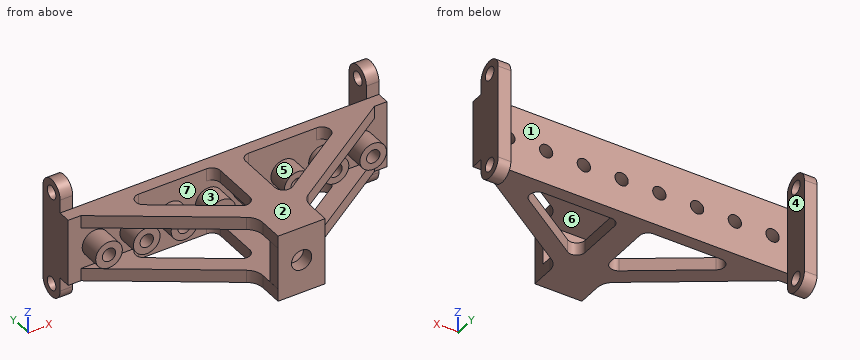
```python
from build123d import *

# Parameters (mm, degrees)
SKETCH1_W            = 70
SKETCH1_H            = 16
SKETCH1_R            = 1.5875
BOSS_EXTRUDE1_DEPTH  = 3
BOSS_EXTRUDE6_DEPTH  = 3
BOSS_EXTRUDE9_START  = -3
BOSS_EXTRUDE9_DEPTH  = 3
SKETCH7_W            = 11.213160903
SKETCH7_H            = 16
SKETCH7_R            = 2.413
BOSS_EXTRUDE10_DEPTH = 3
SKETCH10_R           = 1.5875
BOSS_EXTRUDE11_DEPTH = 3
BOSS_EXTRUDE12_START = 3
SKETCH11_R           = 1.5875
BOSS_EXTRUDE12_DEPTH = 3
SKETCH12_R           = 3.175
SKETCH12_R_2         = 1.5875
BOSS_EXTRUDE13_DEPTH = 5


with BuildPart() as part:
    # Sketch1 → Boss-Extrude1 (new body)
    with BuildSketch(Plane(origin=(0, 0, 0), x_dir=(1, 0, 0), z_dir=(0, 1, 0))):
        Rectangle(SKETCH1_W, SKETCH1_H)
        with Locations(Location((-4.5, 0, 0), (0, 0, 270))):
            Circle(SKETCH1_R, mode=Mode.SUBTRACT)
        with Locations(Location((4.5, 0, 0), (0, 0, 270))):
            Circle(SKETCH1_R, mode=Mode.SUBTRACT)
        with Locations(Location((13.5, 0, 0), (0, 0, 270))):
            Circle(SKETCH1_R, mode=Mode.SUBTRACT)
        with Locations(Location((22.5, 0, 0), (0, 0, 270))):
            Circle(SKETCH1_R, mode=Mode.SUBTRACT)
        with Locations(Location((31.5, 0, 0), (0, 0, 270))):
            Circle(SKETCH1_R, mode=Mode.SUBTRACT)
        with Locations(Location((-13.5, 0, 0), (0, 0, 270))):
            Circle(SKETCH1_R, mode=Mode.SUBTRACT)
        with Locations(Location((-22.5, 0, 0), (0, 0, 270))):
            Circle(SKETCH1_R, mode=Mode.SUBTRACT)
        with Locations(Location((-31.5, 0, 0), (0, 0, 270))):
            Circle(SKETCH1_R, mode=Mode.SUBTRACT)
    extrude(amount=-BOSS_EXTRUDE1_DEPTH)

    # Sketch3 → Boss-Extrude6 (add)
    with BuildSketch(Plane(origin=(0, 0, -8), x_dir=(-1, 0, 0), z_dir=(0, 0, -1))):
        with BuildLine():
            ThreePointArc((-7.390034655, -21.480696382), (-6.086556875, -22.920616292), (-5.615003916, -24.804776975))
            Line((-5.615003916, -24.804776975), (-5.615003916, -30.4))
            Line((-5.615003916, -30.4), (5.615003916, -30.4))
            Line((5.615003916, -30.4), (5.615003916, -24.804776975))
            ThreePointArc((5.615003916, -24.804776975), (6.086556875, -22.920616292), (7.390034655, -21.480696382))
            Line((7.390034655, -21.480696382), (35, -3))
            Line((35, -3), (35, 0))
            Line((35, 0), (-35, 0))
            Line((-35, 0), (-35, -3))
            Line((-35, -3), (-7.390034655, -21.480696382))
        make_face()
        with BuildLine():
            Line((-6.11248463, -17.522461887), (-22.337839864, -6.662040296))
            ThreePointArc((-22.337839864, -6.662040296), (-23.139001046, -4.418656983), (-21.225355233, -3))
            Line((-21.225355233, -3), (-5, -3))
            ThreePointArc((-5, -3), (-3.585786438, -3.585786438), (-3, -5))
            Line((-3, -5), (-3, -15.860421591))
            ThreePointArc((-3, -15.860421591), (-4.057919659, -17.624645111), (-6.11248463, -17.522461887))
        make_face(mode=Mode.SUBTRACT)
        with BuildLine():
            Line((3, -15.860421591), (3, -5))
            ThreePointArc((3, -5), (3.585786438, -3.585786438), (5, -3))
            Line((5, -3), (21.225355233, -3))
            ThreePointArc((21.225355233, -3), (23.139001046, -4.418656983), (22.337839864, -6.662040296))
            Line((22.337839864, -6.662040296), (6.11248463, -17.522461887))
            ThreePointArc((6.11248463, -17.522461887), (4.057919659, -17.624645111), (3, -15.860421591))
        make_face(mode=Mode.SUBTRACT)
    extrude(amount=-BOSS_EXTRUDE6_DEPTH)

    # Sketch6 → Boss-Extrude9 (add)
    with BuildSketch(Plane.XY.offset(8).offset(BOSS_EXTRUDE9_START)):
        with BuildLine():
            ThreePointArc((-7.390034655, -21.480696382), (-6.086556875, -22.920616292), (-5.615003916, -24.804776975))
            Line((-5.615003916, -24.804776975), (-5.615003916, -30.4))
            Line((-5.615003916, -30.4), (5.615003916, -30.4))
            Line((5.615003916, -30.4), (5.615003916, -24.804776975))
            ThreePointArc((5.615003916, -24.804776975), (6.086556875, -22.920616292), (7.390034655, -21.480696382))
            Line((7.390034655, -21.480696382), (35, -3))
            Line((35, -3), (35, 0))
            Line((35, 0), (-35, 0))
            Line((-35, 0), (-35, -3))
            Line((-35, -3), (-7.390034655, -21.480696382))
        make_face()
        with BuildLine():
            Line((-6.11248463, -17.522461887), (-22.337839864, -6.662040296))
            ThreePointArc((-22.337839864, -6.662040296), (-23.139001046, -4.418656983), (-21.225355233, -3))
            Line((-21.225355233, -3), (-5, -3))
            ThreePointArc((-5, -3), (-3.585786438, -3.585786438), (-3, -5))
            Line((-3, -5), (-3, -15.860421591))
            ThreePointArc((-3, -15.860421591), (-4.057919659, -17.624645111), (-6.11248463, -17.522461887))
        make_face(mode=Mode.SUBTRACT)
        with BuildLine():
            Line((3, -15.860421591), (3, -5))
            ThreePointArc((3, -5), (3.585786438, -3.585786438), (5, -3))
            Line((5, -3), (21.225355233, -3))
            ThreePointArc((21.225355233, -3), (23.139001046, -4.418656983), (22.337839864, -6.662040296))
            Line((22.337839864, -6.662040296), (6.11248463, -17.522461887))
            ThreePointArc((6.11248463, -17.522461887), (4.057919659, -17.624645111), (3, -15.860421591))
        make_face(mode=Mode.SUBTRACT)
    extrude(amount=BOSS_EXTRUDE9_DEPTH)

    # Sketch7 → Boss-Extrude10 (add)
    with BuildSketch(Plane.XZ.offset(30.4)):
        with Locations((0.008423464, 0)):
            Rectangle(SKETCH7_W, SKETCH7_H)
        Circle(SKETCH7_R, mode=Mode.SUBTRACT)
    extrude(amount=-BOSS_EXTRUDE10_DEPTH)

    # Sketch10 → Boss-Extrude11 (add)
    with BuildSketch(Plane(origin=(35, 0, 0), x_dir=(0, 0, -1), z_dir=(1, 0, 0))):
        with BuildLine():
            Line((-11.175, 0), (-8, 0))
            Line((-8, 0), (-8, -3))
            Line((-8, -3), (8, -3))
            Line((8, -3), (8, 0))
            Line((8, 0), (11.175, 0))
            ThreePointArc((11.175, 0), (14.35, 3.175), (11.175, 6.35))
            Line((11.175, 6.35), (-11.175, 6.35))
            ThreePointArc((-11.175, 6.35), (-14.35, 3.175), (-11.175, 0))
        make_face()
        with Locations(Location((11.175, 3.175, 0), (0, 0, 180))):
            Circle(SKETCH10_R, mode=Mode.SUBTRACT)
        with Locations((-11.175, 3.175)):
            Circle(SKETCH10_R, mode=Mode.SUBTRACT)
    extrude(amount=BOSS_EXTRUDE11_DEPTH)

    # Sketch11 → Boss-Extrude12 (add)
    with BuildSketch(Plane.ZY.offset(35).offset(BOSS_EXTRUDE12_START)):
        with BuildLine():
            Line((-11.175, 0), (-8, 0))
            Line((-8, 0), (-8, -3))
            Line((-8, -3), (8, -3))
            Line((8, -3), (8, 0))
            Line((8, 0), (11.175, 0))
            ThreePointArc((11.175, 0), (14.35, 3.175), (11.175, 6.35))
            Line((11.175, 6.35), (-11.175, 6.35))
            ThreePointArc((-11.175, 6.35), (-14.35, 3.175), (-11.175, 0))
        make_face()
        with Locations(Location((11.175, 3.175, 0), (0, 0, 180))):
            Circle(SKETCH11_R, mode=Mode.SUBTRACT)
        with Locations((-11.175, 3.175)):
            Circle(SKETCH11_R, mode=Mode.SUBTRACT)
    extrude(amount=-BOSS_EXTRUDE12_DEPTH)

    # Sketch12 → Boss-Extrude13 (add)
    # profile 1 of 8: a face of its own
    with BuildSketch(Plane.XZ.offset(3)):
        with Locations(Location((-31.5, 0, 0), (0, 0, 270))):
            Circle(SKETCH12_R)
        with Locations(Location((-31.5, 0, 0), (0, 0, 90))):
            Circle(SKETCH12_R_2, mode=Mode.SUBTRACT)
    # profile 2 of 8: a face of its own
    with BuildSketch(Plane.XZ.offset(3)):
        with Locations(Location((-22.5, 0, 0), (0, 0, 270))):
            Circle(SKETCH12_R)
        with Locations(Location((-22.5, 0, 0), (0, 0, 90))):
            Circle(SKETCH12_R_2, mode=Mode.SUBTRACT)
    # profile 3 of 8: a face of its own
    with BuildSketch(Plane.XZ.offset(3)):
        with Locations(Location((-13.5, 0, 0), (0, 0, 270))):
            Circle(SKETCH12_R)
        with Locations(Location((-13.5, 0, 0), (0, 0, 90))):
            Circle(SKETCH12_R_2, mode=Mode.SUBTRACT)
    # profile 4 of 8: a face of its own
    with BuildSketch(Plane.XZ.offset(3)):
        with Locations(Location((-4.5, 0, 0), (0, 0, 270))):
            Circle(SKETCH12_R)
        with Locations(Location((-4.5, 0, 0), (0, 0, 90))):
            Circle(SKETCH12_R_2, mode=Mode.SUBTRACT)
    # profile 5 of 8: a face of its own
    with BuildSketch(Plane.XZ.offset(3)):
        with Locations(Location((4.5, 0, 0), (0, 0, 270))):
            Circle(SKETCH12_R)
        with Locations(Location((4.5, 0, 0), (0, 0, 90))):
            Circle(SKETCH12_R_2, mode=Mode.SUBTRACT)
    # profile 6 of 8: a face of its own
    with BuildSketch(Plane.XZ.offset(3)):
        with Locations(Location((13.5, 0, 0), (0, 0, 270))):
            Circle(SKETCH12_R)
        with Locations(Location((13.5, 0, 0), (0, 0, 90))):
            Circle(SKETCH12_R_2, mode=Mode.SUBTRACT)
    # profile 7 of 8: a face of its own
    with BuildSketch(Plane.XZ.offset(3)):
        with Locations(Location((22.5, 0, 0), (0, 0, 270))):
            Circle(SKETCH12_R)
        with Locations(Location((22.5, 0, 0), (0, 0, 90))):
            Circle(SKETCH12_R_2, mode=Mode.SUBTRACT)
    # profile 8 of 8: a face of its own
    with BuildSketch(Plane.XZ.offset(3)):
        with Locations(Location((31.5, 0, 0), (0, 0, 270))):
            Circle(SKETCH12_R)
        with Locations(Location((31.5, 0, 0), (0, 0, 90))):
            Circle(SKETCH12_R_2, mode=Mode.SUBTRACT)
    extrude(amount=BOSS_EXTRUDE13_DEPTH)


solid = part.part
```
Design review of the part built by this model. Coordinates are the model's own, in mm. Face numbers are marked on the shaded views. A direction names the side the tool comes from. Coordinates: 2 decimals unless noted, no trailing zeros. Order: outer loops, then holes, each group sorted by start corner. A loop starts at its lowest first (then second) coordinate and runs counter-clockwise, first axis right, second up. Notation, with made-up numbers: (57, -28) -> (72, -28) arc R25 ccw to (72, -7) -> close; hole circle Ø8 at (-25.75, 81). An arc over 180 degrees is marked (long way). One line per item, written item: value. Start each with the question number.
Q1. Take a section at B-B, the plane x = 31.5. State the section outline as (y, z) points (1 decimal).
Q2. Insertion check: pin 1 Ø10 at (x, y) = (-3.5, -0.5) entering from -Z; pin 2 Ø2.5 at (x, z) = (-4.5, 0) entering from +Y; pin 3 Ø6 at (x, y) = (22.5, -17.5) entering from -Z; pin 4 Ø6 at (x, z) = (16.5, 1) entering from +Y. Each pin has a flat end and moves straight along its axis. Give the tip position at first contact, or say it passes through.
Q3. For probe 1 along X at (y, z) = (5.5, -7.75); probe 2 along Y at (x, z) = (12, -3.25); probe 3 along Z at (x, y) = (-31, -4), list the stretches that pass through material, from the lowest coordinate up.
Q4. Take a section at A-A, the plane z = -7. State the section outline as (x, y) points (3 decimals), then the cut area to 3 significant figures.
Q5. Mouldability with a two-part tool opening along Y and no side actions: class the marked faces 1, 2 and 3 as pulls with the +Y half, pulls with the -Y half, needs draft (parallel to the pull), parting line crosses it, or undercut.
Q6. Tool access review of the marked faces 4, 5, 6 and 7: name each direction out of +Z, -Z, +X, -X, +Y, -Y from which nothing blocks a thin tool from reaching the whole face with its end or side.
Q7. Take a section at C-C, the plane y = -1. Give the number of separate pieces and of enclosed holes in the cut face, then the cut area to 3 significant figures.
Values follow:
1. outline: (-8, -3.2) -> (-3, -3.2) -> (-3, -5) -> (-5.3, -5) -> (-5.3, -8) -> (0, -8) -> (0, -1.6) -> (-8, -1.6) -> close; (-8, 1.6) -> (0, 1.6) -> (0, 8) -> (-5.3, 8) -> (-5.3, 5) -> (-3, 5) -> (-3, 3.2) -> (-8, 3.2) -> close
2. pin 1: stops at z = -8
2. pin 2: stops at y = -27.4
2. pin 3: passes through
2. pin 4: stops at y = 0
3. probe 1: x = -38 to -35, 35 to 38
3. probe 2: y = -3 to 0
3. probe 3: z = -8 to -5, -3.14 to -1.51, 1.51 to 3.14, 5 to 8
4. outline: (-38, -3) -> (-35, -3) -> (-7.39, -21.481) arc R4 cw to (-5.615, -24.805) -> (-5.615, -30.4) -> (5.615, -30.4) -> (5.615, -24.805) arc R4 cw to (7.39, -21.481) -> (35, -3) -> (38, -3) -> (38, 6.35) -> (35, 6.35) -> (35, 0) -> (-35, 0) -> (-35, 6.35) -> (-38, 6.35) -> close; hole (-22.338, -6.662) -> (-6.112, -17.522) arc R2 ccw to (-3, -15.86) -> (-3, -5) arc R2 ccw to (-5, -3) -> (-21.225, -3) arc R2 ccw to start; hole (3, -15.86) arc R2 ccw to (6.112, -17.522) -> (22.338, -6.662) arc R2 ccw to (21.225, -3) -> (5, -3) arc R2 ccw to (3, -5) -> close
4. area: 765 mm2
5. face 1: pulls with the +Y half
5. face 2: needs draft
5. face 3: undercut
6. face 4: +Z, -Z, +Y
6. face 5: -Y
6. face 6: +X, -X
6. face 7: none
7. separate pieces: 1
7. enclosed holes: 8
7. area: 1,150 mm2
